Here's how the part is built. I have some questions about the finished solid (model axes, mm). A direction names the side the tool comes from. Round coordinates to 2 decimals unless told otherwise and drop trailing zeros. Write each loop counter-clockwise with the first axis right and the second up, starting at its lowest first coordinate (ties: lowest second). Pieces come first, ordered by that corner, then holes. Notation, with made-up numbers: (65, 55) - (79, 55) arc R31 cw to (79, 85) - close; hole circle Ø3 at (-18, 12.25). An arc over 180 degrees is marked (long way). Write item = value, one per line. Start each with the question number.
Item 1: If we section it at B-B (y = -14.16): Please give me the cut outline in (x, z).
Item 2: Thinking about a two-plate mould opening in X: for faces 4 (the face through (3, 0, 2)), 5 (the face through (21.774, 5.204, 1.972)), 6 (the face through (10.86, -16.75, 1.97)), which applies, pulls with the +X half, pulls with the -X half, needs draft (parallel to the pull), parting line crosses it, or undercut?
Item 3: If we section it at C-C (z = 3.5): Please give me the cut outline in (x, y), and give its area (3 significant figures).
Item 4: If we section it at D-D (y = -6): Please give me the cut outline in (x, z).
Item 5: If I drill on line 1 along Y through (x, z) = (11.43, 2.05); line 2 along X through (y, z) = (-9.5, 2.3); line 3 along X through (y, z) = (-11.75, 0.5), over which ranges is the centre line in solid material (lowest first)? Write a range as [from, to].
Item 6: If we section it at A-A (x = 11.43): Please give me the cut outline in (y, z), and give its area (3 significant figures).
Item 7: Which directions (+Z, -Z, +X, -X, +Y, -Y) give clear straight access to the entire face, cutting with the end or side of a thin tool? Please do faces 1 (the face through (5.08, -8, 2)), 2 (the face through (11, -4, 0)), 3 (the face through (17.78, -8, 2)).
Item 8: For P1, Ø1.5, axis at x = 11, y = -14.5, coming from the +Z side; P2, Ø1.2, axis at x = 19.5, z = 1, coming from the -Y side; P3, Ø2, axis at y = -10, z = 2.5, coming from the -X side, each with a flat end and sliding along its axis, tell me the tip position at first contact or that it passes through.
```python
from build123d import *

# Parameters (mm, degrees)
SKETCH1_R           = 2.65
BOSS_EXTRUDE1_DEPTH = 4


with BuildPart() as part:
    # Sketch1 → Boss-Extrude1 (new body)
    with BuildSketch(Plane.XY):
        with BuildLine():
            Line((0, 0), (5.08, 0))
            Line((5.08, 0), (5.08, -16.7))
            ThreePointArc((5.08, -16.7), (6.195923164, -19.394076836), (8.89, -20.51))
            Line((8.89, -20.51), (13.97, -20.51))
            ThreePointArc((13.97, -20.51), (16.664076836, -19.394076836), (17.78, -16.7))
            Line((17.78, -16.7), (17.78, 0))
            Line((17.78, 0), (22.86, 0))
            Line((22.86, 0), (22.86, 2.54))
            ThreePointArc((22.86, 2.54), (21.744076836, 5.234076836), (19.05, 6.35))
            Line((19.05, 6.35), (3.81, 6.35))
            ThreePointArc((3.81, 6.35), (1.115923164, 5.234076836), (0, 2.54))
            Line((0, 2.54), (0, 0))
        make_face()
        with Locations((11.43, -14.16)):
            Circle(SKETCH1_R, mode=Mode.SUBTRACT)
    extrude(amount=BOSS_EXTRUDE1_DEPTH)


solid = part.part
```
Reply:
q1.outline = (5.08, 0) - (8.78, 0) - (8.78, 4) - (5.08, 4) - close; (14.08, 0) - (17.78, 0) - (17.78, 4) - (14.08, 4) - close
q2.face_4 = needs draft
q2.face_5 = pulls with the +X half
q2.face_6 = undercut
q3.outline = (0, 0) - (5.08, 0) - (5.08, -16.7) arc R3.81 ccw to (8.89, -20.51) - (13.97, -20.51) arc R3.81 ccw to (17.78, -16.7) - (17.78, 0) - (22.86, 0) - (22.86, 2.54) arc R3.81 ccw to (19.05, 6.35) - (3.81, 6.35) arc R3.81 ccw to (0, 2.54) - close; hole circle Ø5.3 at (11.43, -14.16)
q3.area = 371 mm2
q4.outline = (5.08, 0) - (17.78, 0) - (17.78, 4) - (5.08, 4) - close
q5.line_1 = [-20.51, -16.81], [-11.51, 6.35]
q5.line_2 = [5.08, 17.78]
q5.line_3 = [5.08, 10.33], [12.53, 17.78]
q6.outline = (-20.51, 0) - (-16.81, 0) - (-16.81, 4) - (-20.51, 4) - close; (-11.51, 0) - (6.35, 0) - (6.35, 4) - (-11.51, 4) - close
q6.area = 86.2 mm2
q7.face_1 = +Z, -Z, -X, -Y
q7.face_2 = -Z, +X, -X, +Y, -Y
q7.face_3 = +Z, -Z, +X, -Y
q8.P1 = through
q8.P2 = 0
q8.P3 = 5.08
